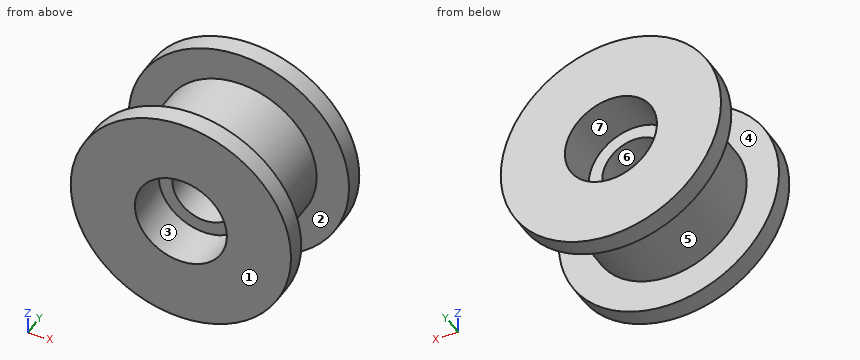
Autodesk Inventor part; units mm, degrees
ref_plane "YZ Plane" through (0, 0, 0) normal (1, 0, 0) x (0, 1, 0)
ref_plane "XZ Plane" through (0, 0, 0) normal (0, 1, 0) x (-1, 0, 0)
ref_plane "XY Plane" through (0, 0, 0) normal (0, 0, 1) x (1, 0, 0)
sketch "Sketch1" plane through (0, 0, 0) normal (0, 1, 0) x (-1, 0, 0)
  circle A0 centre (0, 0) radius 6
  dimension "d0" = 12
extrude "Extrusion1" add sketch "Sketch1" along normal mid plane 7
sketch "Sketch2" plane through (0, 3.5, 0) normal (0, 1, 0) x (1, 0, 0)
  circle A0 centre (0, 0) radius 8.5
  dimension "d3" = 17
extrude "Extrusion2" add sketch "Sketch2" along normal blind 1.5
sketch "Sketch3" plane through (0, -3.5, 0) normal (0, -1, 0) x (1, 0, 0)
  circle A0 centre (0, 0) radius 8.5
  dimension "d8" = 17
extrude "Extrusion3" add sketch "Sketch3" along normal blind 1.5
sketch "Sketch4" plane through (0, 5, 0) normal (0, 1, 0) x (1, 0, 0)
  circle A0 centre (0, 0) radius 2.5
  dimension "d9" = 5
extrude "Extrusion4" cut sketch "Sketch4" against normal up to next
sketch "Sketch8" plane through (0, 5, 0) normal (0, 1, 0) x (1, 0, 0)
  circle A0 centre (0, 0) radius 3.55
  dimension "d12" = 7.1
extrude "Extrusion5" cut sketch "Sketch8" against normal blind 3.5
sketch "Sketch9" plane through (0, -5, 0) normal (0, -1, 0) x (1, 0, 0)
  circle A0 centre (0, 0) radius 3.55
  dimension "d15" = 7.1
extrude "Extrusion6" cut sketch "Sketch9" against normal blind 3.5
properties part number "Катушка" material "Polypropylene"
Design review of the part built by this model. Coordinates are the model's own, in mm. Face numbers are marked on the shaded views. A direction names the side the tool comes from. Round coordinates to 2 decimals unless told otherwise and drop trailing zeros. Write each loop counter-clockwise with the first axis right and the second up, starting at its lowest first coordinate (ties: lowest second). Pieces come first, ordered by that corner, then holes.
Item 1: We need section A-A on z = 0. Write out the cut boundary in (x, y), and give its area (3 significant figures).
Item 2: We need section C-C on y = 1. Write out the cut boundary in (x, z), and give its area (3 significant figures).
Item 3: For the marked faces 1, 2 and 3, list the 3-axis set-ups (+Z, -Z, +X, -X, +Y, -Y) from which the entire face can be reached by the end or side of a thin tool; tool diameter is ignored.
Item 4: Clearance check with flat-ended pins moving along their axes: pin 1 Ø4 at (x, y) = (3, 3.5) entering from +Z; pin 2 Ø2 at (y, z) = (-1, -1) entering from -X; pin 3 Ø1 at (x, y) = (3.5, -2.5) entering from +Z. State where each tip first meets the part, or that it passes through.
Item 5: For probe 1 along X at (y, z) = (3.9, 0); probe 2 along Z at (x, y) = (0, 0.85); probe 3 along Y at (x, z) = (-0.5, -6.75), list the stretches that pass through material, from the lowest coordinate up.
Item 6: We need section B-B on x = 0. Write out the cut boundary in (y, z), and give its area (3 significant figures).
Item 7: We need section D-D on x = -3.25. Write out the cut boundary in (y, z), and give its area (3 significant figures).
Item 8: The part is to be moulded in two halves that separate along X. For the marked faces 4, 5, 6 and 7, say which applies: +X half, -X half, draft (parallel to the pull), parting line (faces both ways), or undercut.
Returned:
1. outline: (-8.5, -5) - (-3.55, -5) - (-3.55, -1.5) - (-2.5, -1.5) - (-2.5, 1.5) - (-3.55, 1.5) - (-3.55, 5) - (-8.5, 5) - (-8.5, 3.5) - (-6, 3.5) - (-6, -3.5) - (-8.5, -3.5) - close; (2.5, -1.5) - (3.55, -1.5) - (3.55, -5) - (8.5, -5) - (8.5, -3.5) - (6, -3.5) - (6, 3.5) - (8.5, 3.5) - (8.5, 5) - (3.55, 5) - (3.55, 1.5) - (2.5, 1.5) - close
1. area: 70.3 mm2
2. outline: circle Ø12 at (0, 0); hole circle Ø5 at (0, 0)
2. area: 93.5 mm2
3. face 1: +Z, -Z, +X, -X, -Y
3. face 2: none
3. face 3: -Y
4. pin 1: stops at z = 8.44
4. pin 2: stops at x = -6
4. pin 3: stops at z = 5.2
5. probe 1: x = -8.5 to -3.55, 3.55 to 8.5
5. probe 2: z = -6 to -2.5, 2.5 to 6
5. probe 3: y = -5 to -3.5, 3.5 to 5
6. outline: (-5, -8.5) - (-3.5, -8.5) - (-3.5, -6) - (3.5, -6) - (3.5, -8.5) - (5, -8.5) - (5, -3.55) - (1.5, -3.55) - (1.5, -2.5) - (-1.5, -2.5) - (-1.5, -3.55) - (-5, -3.55) - close; (-5, 3.55) - (-1.5, 3.55) - (-1.5, 2.5) - (1.5, 2.5) - (1.5, 3.55) - (5, 3.55) - (5, 8.5) - (3.5, 8.5) - (3.5, 6) - (-3.5, 6) - (-3.5, 8.5) - (-5, 8.5) - close
6. area: 70.3 mm2
7. outline: (-5, -7.85) - (-3.5, -7.85) - (-3.5, -5.04) - (3.5, -5.04) - (3.5, -7.85) - (5, -7.85) - (5, -1.43) - (1.5, -1.43) - (1.5, 1.43) - (5, 1.43) - (5, 7.85) - (3.5, 7.85) - (3.5, 5.04) - (-3.5, 5.04) - (-3.5, 7.85) - (-5, 7.85) - (-5, 1.43) - (-1.5, 1.43) - (-1.5, -1.43) - (-5, -1.43) - close
7. area: 97.7 mm2
8. face 4: draft
8. face 5: parting line
8. face 6: undercut
8. face 7: undercut
